from build123d import *

# Parameters (mm, degrees)
BOSS_EXTRUDE1_DEPTH     = 38.1
SKETCH2_R               = 6.35
CUT_EXTRUDE1_DEPTH      = 277.034883433
ADVANCEDHOLE3_OUTLINE_R = 9.525
ADVANCEDHOLE3_DEPTH     = 38.1
SKETCH21_R              = 6.35
CUT_EXTRUDE2_DEPTH      = 35.56
SKETCH23_R              = 6.35
BOSS_EXTRUDE2_DEPTH     = 12.7


# Read off the part's stored shape, not the designer's step: AdvancedHole3
with BuildPart() as part:
    # Sketch1 → Boss-Extrude1 (new body)
    with BuildSketch(Plane.XY):
        with BuildLine():
            Line((0, 0), (0, 203.013094366))
            ThreePointArc((0, 203.013094366), (50.8, 253.813094366), (101.6, 203.013094366))
            Line((101.6, 203.013094366), (101.6, 0))
            ThreePointArc((101.6, 0), (50.8, -50.8), (0, 0))
        make_face()
    extrude(amount=BOSS_EXTRUDE1_DEPTH)

    # Sketch2 → Cut-Extrude1 (cut, through all)
    with BuildSketch(Plane(origin=(101.6, 0, 0), x_dir=(0, 0, -1), z_dir=(1, 0, 0))):
        with Locations(Location((-19.05, 101.506547183, 0), (0, 0, 90))):
            Circle(SKETCH2_R)
    extrude(amount=-CUT_EXTRUDE1_DEPTH, mode=Mode.SUBTRACT)

    # AdvancedHole3 outline → AdvancedHole3 (cut)
    with BuildSketch(Plane.XY):
        with Locations((50.8, 203.013094366)):
            Circle(ADVANCEDHOLE3_OUTLINE_R)
        with Locations((50.8, 0)):
            Circle(ADVANCEDHOLE3_OUTLINE_R)
    extrude(amount=ADVANCEDHOLE3_DEPTH, mode=Mode.SUBTRACT)

    # Sketch21 → Cut-Extrude2 (cut)
    with BuildSketch(Plane.XY.offset(38.1)):
        with Locations((50.8, 50.706547183)):
            Circle(SKETCH21_R)
        with Locations((50.8, 152.213094366)):
            Circle(SKETCH21_R)
    extrude(amount=-CUT_EXTRUDE2_DEPTH, mode=Mode.SUBTRACT)

    # Sketch23 → Boss-Extrude2 (add)
    with BuildSketch(Plane.XY.offset(38.1)):
        with Locations((50.8, 101.506547183)):
            Circle(SKETCH23_R)
    extrude(amount=BOSS_EXTRUDE2_DEPTH)


solid = part.part
Design review of the part built by this model. Coordinates are the model's own, in mm. A direction names the side the tool comes from. Give positions to 0.01 mm unless a question says otherwise; leave off trailing zeros. Order: outer loops, then holes, each group sorted by start corner. A loop starts at its lowest first (then second) coordinate and runs counter-clockwise, first axis right, second up. Notation, with made-up numbers: (-3.5, 15.5) - (26.5, 15.5) arc R15 ccw to (26.5, 42.5) - close; hole circle Ø7 at (-7.75, 55). An arc over 180 degrees is marked (long way). Write item = value, one per line. Start each with the question number.
Q1. We need section A-A on x = 50.8. State the section outline as (y, z) points (3 decimals), plus the area to 3 significant figures.
Q2. Clearance check with flat-ended pins moving along their axes: pin 1 Ø12 at (x, z) = (67, 32) entering from +Y; pin 2 Ø14.5 at (y, z) = (101.51, 19.05) entering from +X; pin 3 Ø6.5 at (x, y) = (52, 51.5) entering from +Z; pin 4 Ø6 at (x, y) = (37, -7) entering from +Z. State where each tip first meets the part, or that it passes through.
Q3. We need section B-B on z = 19.05. State the section outline as (x, y) points (3 decimals).
Q4. We need section C-C on y = 209. State the section outline as (x, z) points, plus the area to 3 significant figures.
Q5. We need section D-D on x = 25.5. State the section outline as (y, z) points, plus the area to 3 significant figures.
Q6. Mouldability with a two-part tool opening along Y and no side actions: class faces 3 (the face through (51.917, -50.788, 18.783)), 4 (the face through (52, 104, 0)), 5 (the face through (51, 152, 2.54)) as released by +Y, released by -Y, zero draft, split by the parting line, or undercut.
Q7. To check wall thickness, follow L1, parallel to Y at x = 50.8, z = 10 (3 decimals); L2, parallel to Y at x = 50, z = 26; L3, parallel to X at y = 152, z = 24. State the ranges of each line that lie inside material, in increasing order. Write a range as from..to.
Q8. Tool access review of faces 1 (the face through (101.6, 103, 27)), 2 (the face through (56.666, 149.781, 20.569)): name each direction out of +Z, -Z, +X, -X, +Y, -Y from which nothing blocks a thin tool from reaching the whole face with its end or side.
Working result:
q1.outline = (-50.8, 0) - (-9.525, 0) - (-9.525, 38.1) - (-50.8, 38.1) - close; (9.525, 0) - (193.488, 0) - (193.488, 38.1) - (158.563, 38.1) - (158.563, 2.54) - (145.863, 2.54) - (145.863, 38.1) - (107.857, 38.1) - (107.857, 50.8) - (95.157, 50.8) - (95.157, 38.1) - (57.057, 38.1) - (57.057, 2.54) - (44.357, 2.54) - (44.357, 38.1) - (9.525, 38.1) - close; (212.538, 0) - (253.813, 0) - (253.813, 38.1) - (212.538, 38.1) - close; hole circle Ø12.7 at (101.507, 19.05)
q1.area = 9,290 mm²
q2.pin_1 = 252.78
q2.pin_2 = 101.6
q2.pin_3 = 2.54
q2.pin_4 = 38.1
q3.outline = (0, 0) arc R50.8 ccw to (101.6, 0) - (101.6, 95.157) - (0, 95.157) - close; (0, 107.857) - (101.6, 107.857) - (101.6, 203.013) arc R50.8 ccw to (0, 203.013) - close; hole circle Ø19.05 at (50.8, 0); hole circle Ø19.05 at (50.8, 203.013); hole circle Ø12.7 at (50.8, 50.707); hole circle Ø12.7 at (50.8, 152.213)
q4.outline = (0.35, 0) - (43.39, 0) - (43.39, 38.1) - (0.35, 38.1) - close; (58.21, 0) - (101.25, 0) - (101.25, 38.1) - (58.21, 38.1) - close
q4.area = 3,280 mm²
q5.outline = (-44.05, 0) - (247.06, 0) - (247.06, 38.1) - (-44.05, 38.1) - close; hole circle Ø12.7 at (101.51, 19.05)
q5.area = 11,000 mm²
q6.face_3 = released by -Y
q6.face_4 = zero draft
q6.face_5 = undercut
q7.L1 = -50.8..-9.525, 9.525..44.357, 57.057..145.863, 158.563..193.488, 212.538..253.813
q7.L2 = -50.79..-9.49, 9.49..44.41, 57.01..145.91, 158.51..193.52, 212.5..253.81
q7.L3 = 0..44.45, 57.15..101.6
q8.face_1 = +Z, -Z, +X, +Y, -Y
q8.face_2 = +Z
